from build123d import *

# Parameters (mm, degrees)
F1_DEPTH = 12.7
F3_D     = 6.35


with BuildPart() as f1:
    # F0 (on Front) → F1 (new body)
    with BuildSketch(Plane.XZ):
        Polygon((-30.378454, 28.231527), (-30.378454, -174.968473), (-4.978454, -174.968473), (-4.978454, 28.231527), (7.721546, 28.231527), (7.721546, 53.631527), (-43.078454, 53.631527), (-43.078454, 28.231527), align=None)
    extrude(amount=-F1_DEPTH)

    # F3 (through all)
    with Locations(Plane.XZ):
        with Locations((-17.678454, -162.268473)):
            Hole(F3_D / 2)


solid = f1.part
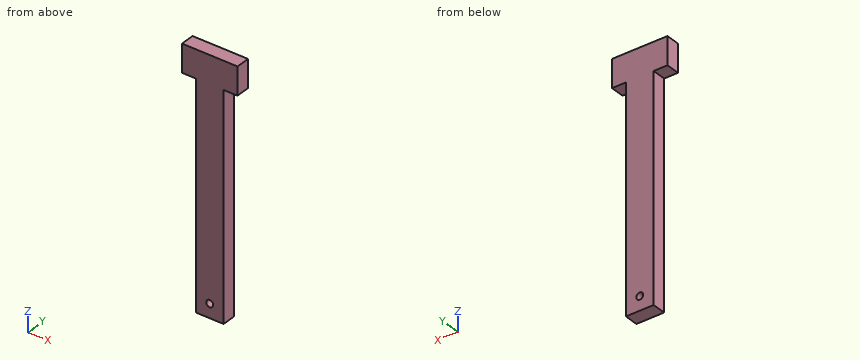
Read the model definition and answer for the solid it produces. Units are mm, in the model's axes. Round coordinates to 2 decimals unless told otherwise and drop trailing zeros. Loops run counter-clockwise (first coordinate to the right, second up) from the corner with the lowest first, then second, coordinate; pieces in that order, holes last. Notation, with made-up numbers: (-21.75, 85.25) - (3.25, 85.25) arc R27 ccw to (3.25, 120.25) - close; hole circle Ø7 at (-29.75, 85.5). An arc over 180 degrees is marked (long way). One line per question, with ' | ' between items. Start each with the question number.
Q1. Find the intervals of material crossed by L1, parallel to X at y = 10.75, z = -162; L2, parallel to X at y = 8.25, z = -3; L3, parallel to Z at x = -34, y = 7.75, in increasing order.
Q2. Section C-C on z = 21.5 is taken. Give the vertices of the cut face in (x, y).
Q3. Flat-ended cylindrical pins translate along their axes: pin 1 (1.5 mm diameter, centred on y = 2.5, z = -7, fed in from -X); pin 2 (1 mm diameter, centred on x = -2.5, z = -1, fed in from +Y); pin 3 (6.5 mm diameter, centred on x = -37.5, y = 5, fed in from -Z). Find the tip coordinate at first contact, or state that the pin passes through.
Q4. Section A-A on y = 3 is taken. Give the vertices of the cut face in (x, z) (3 decimals).
Q5. Section B-B on x = -2 is taken. Give the vertices of the cut face in (y, z), plus the area to 3 significant figures.
Established:
1) L1: -30.38 to -20.84, -14.51 to -4.98 | L2: -30.38 to -4.98 | L3: 28.23 to 53.63
2) outline: (-30.38, 0) - (-4.98, 0) - (-4.98, 12.7) - (-30.38, 12.7) - close
3) pin 1: x = -30.38 | pin 2: through | pin 3: z = 28.23
4) outline: (-43.078, 28.232) - (-30.378, 28.232) - (-30.378, -174.968) - (-4.978, -174.968) - (-4.978, 28.232) - (7.722, 28.232) - (7.722, 53.632) - (-43.078, 53.632) - close; hole circle Ø6.35 at (-17.678, -162.268)
5) outline: (0, 28.23) - (12.7, 28.23) - (12.7, 53.63) - (0, 53.63) - close | area: 323 mm²
